Autodesk Inventor part; units mm, degrees
ref_plane "YZ Plane" through (0, 0, 0) normal (1, 0, 0) x (0, 1, 0)
ref_plane "XZ Plane" through (0, 0, 0) normal (0, 1, 0) x (-1, 0, 0)
ref_plane "XY Plane" through (0, 0, 0) normal (0, 0, 1) x (1, 0, 0)
sketch "Sketch1" plane through (0, 0, 0) normal (0, 1, 0) x (-1, 0, 0)
  line L0 (0, 0) -> (90, 0)
  line L1 (90, 0) -> (90, -55.8)
  line L2 (90, -55.8) -> (0, -55.8)
  line L3 (0, -55.8) -> (0, 0)
  ellipse E0 centre (45, -27.9) end of major axis (0, -27.9) minor radius 38.6219 (13.883, -55.8) -> (13.883, 0) ccw
  line L4 (64.8234, -39.45) -> (22.5234, -39.45)
  line L5 (22.5234, -39.45) -> (22.5234, -48.75)
  line L6 (22.5234, -48.75) -> (64.8234, -48.75)
  line L7 (64.8234, -48.75) -> (64.8234, -39.45)
  line L8 (64.8234, -19.35) -> (22.5234, -19.35)
  line L9 (22.5234, -19.35) -> (22.5234, -28.65)
  line L10 (22.5234, -28.65) -> (64.8234, -28.65)
  line L11 (64.8234, -28.65) -> (64.8234, -19.35)
  line L12 (90, -27.9) -> (0, -27.9)
  ellipse E1 centre (12.4971, -44.1) end of major axis (0, -44.1) minor radius 12.8946 (3.6964, -34.945) -> (15.0472, -56.7233) ccw
  line L13 (1.5364, -17.8943) -> (7.2883, -25.7782)
  line L14 (1.5364, -37.9057) -> (7.2883, -30.0218)
  arc A0 (7.2883, -30.0218) -> (7.2883, -25.7782) centre (4.38, -27.9) ccw
  line L15 (85.0982, -24.9854) -> (89.4419, -21.8362)
  line L16 (85.0982, -30.8146) -> (89.4419, -33.9638)
  arc A1 (85.0982, -24.9854) -> (85.0982, -30.8146) centre (87.2113, -27.9) ccw
  ellipse E2 centre (12.4971, -11.7) end of major axis (0, -11.7) minor radius 12.8946 (15.0472, 0.9233) -> (3.6964, -20.855) ccw
  ellipse E3 centre (12.4971, -11.7) end of major axis (0, -11.7) minor radius 12.8946 (22.5234, -19.3972) -> (22.5573, -19.35) ccw
  point P0 (8.8363, -27.9)
  point P1 (81.0782, -27.9)
  point P2 (7.2438, 0)
  point P3 (7.2438, -55.8)
  dimension "d0" = 90
  dimension "d1" = 55.8
  dimension "d3" = 9.3
  dimension "d4" = 9.3
  dimension "d5" = 7.05
  dimension "d6" = 10.8
  dimension "d7" = 3.6
  dimension "d8" = 3.6
extrude "Extrusion1" add sketch "Sketch1" along normal blind 9 contours L0 E0 L15 A1 L12 L11 L8 L9 A0 L13 E2 | E0 L0 | E1 L14 A0 L12 L9 L10 L11 A1 L16 E0 L2 | L2 E0
properties part number "telapak kaki"
Part model, mm, in its own coordinate system. A direction names the side the tool comes from. Give positions to 0.01 mm unless a question says otherwise; leave off trailing zeros. Use CSV: the item, a comma, the result in double quotes.
Item 1: Drill centre lines: probe 1 along X at (y, z) = (6, -28); probe 2 along Z at (x, y) = (-46.5, 5.25); probe 3 along Z at (x, y) = (-55, 3.75). Where is each one in solid material? Low to high.
Taken from the geometry:
probe 1,"x = -83.61 to -64.82, -22.52 to -7.98"
probe 2,"z = -66.5 to -48.75, -39.45 to -28.65, -19.35 to 10.7"
probe 3,"z = -65.56 to -48.75, -39.45 to -28.65, -19.35 to 9.76"
Item 2: Slice it at A-A on x = -35.5. State how many separate pieces and enclosed holes the cut face has, plus the area to 3 significant figures.
Taken from the geometry:
separate pieces,"3"
enclosed holes,"0"
area,"512 mm²"
Item 3: Pin check, flat tips, straight feed: P1, Ø2, axis at x = -78.5, y = 7.5, coming from the -Z side; P2, Ø2.5, axis at y = 6, z = -26.5, coming from the -X side; P3, Ø1.5, axis at y = 7, z = -31, coming from the +X side. Stop position of each tip, or through.
Taken from the geometry:
P1,"stops at z = -54.61"
P2,"stops at x = -84.77"
P3,"stops at x = -6.03"
Item 4: Which spindle directions (+Z, -Z, +X, -X, +Y, -Y) get a long thin tool onto all of the face, cutting with end or side? Do faces 5 (the face through (-4.37, 4.44, -21.78)), 6 (the face through (-11, 4, -55.8)), 7 (the face through (-44, 0, -19)), 8 (the face through (-22.523, 4, -24)), 9 (the face through (-87.24, 4.437, -23.433)). Say none if no direction does.
Taken from the geometry:
face 5,"+X, +Y, -Y"
face 6,"-Z, +X, +Y, -Y"
face 7,"+Z, -Z, +X, -X, -Y"
face 8,"+Y, -Y"
face 9,"-X, +Y, -Y"
Item 5: Pull direction Z, two halves, no side cores. Call faces 1 (the face through (-87.24, 4.437, -32.367)), 2 (the face through (-11, 4, 0)), 3 (the face through (-44, 9, -19)), 4 (the face through (-43, 4, -28.65)): +Z half, -Z half, draft (parallel to the pull), parting line (faces both ways), or undercut.
Taken from the geometry:
face 1,"undercut"
face 2,"+Z half"
face 3,"draft"
face 4,"undercut"
